The listing builds one solid part. Answer for the finished solid, in the listing's coordinates (mm). Face numbers are marked on the shaded views. A direction names the side the tool comes from. Coordinates: 2 decimals unless noted, no trailing zeros. Order: outer loops, then holes, each group sorted by start corner. A loop starts at its lowest first (then second) coordinate and runs counter-clockwise, first axis right, second up. Notation, with made-up numbers: M -6,43.5 L 1,43.5 A30 ccw 1,80.5 Z; hole C -20.75,6 d5. An arc over 180 degrees is marked long. One line per item, written item: value. Start each with the question number.
Q1. The part is cut by section C-C on y = 13.5. Give the vertices of the cut face in (x, z), then the cut area to 3 significant figures.
Q2. The part is cut by section A-A on z = -27. Give the vertices of the cut face in (x, y) (3 decimals), then the cut area to 3 significant figures.
Q3. Each of these flat-tipped pins is pushed along its axis until it touches: pin 1 Ø3 at (x, z) = (-5, -5) entering from +Y; pin 2 Ø3.5 at (y, z) = (7, -26) entering from +X; pin 3 Ø1.5 at (y, z) = (4.5, -25) entering from -X; pin 4 Ø7 at (x, z) = (-4.5, -21) entering from +Y. Where does it stop, or does it pass through?
Q4. Determine the mould class of the marked faces 1, 2, 3 and 4 for opening direction X: pulls with the +X half, pulls with the -X half, needs draft (parallel to the pull), parting line crosses it, or undercut.
Q5. For the marked faces 5, 6 and 7, determine the directions among +Z, -Z, +X, -X, +Y, -Y from which every point of the face is accessible in a straight line to the end or side of a thin tool.
Q6. The part is cut by section B-B on x = -5. Give the vertices of the cut face in (y, z), then the cut area to 3 significant figures.
Q7. Straight lines are drawn through the part: line 1 along Z through (x, y) = (-43, 1.1); line 2 along X through (y, z) = (13.25, -19.5); line 3 along X through (y, z) = (1.25, -30). For each, find the intervals that lie inside material, in ascending order. Write a range as [from, to].
Q8. The part is cut by section D-D on z = -5. Give the vertices of the cut face in (x, y), then the cut area to 3 significant figures.
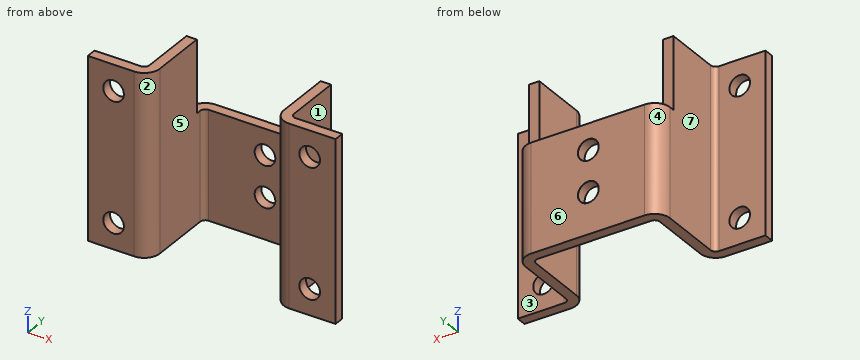
```python
from build123d import *

# Parameters (mm, degrees)
BASE_FLANGE1_DEPTH                 = 35
SKETCH6_W                          = 28
SKETCH6_H                          = 14
CUT_EXTRUDE1_DEPTH                 = 4
F_4_0_4_DIAMETER_HOLE1_D           = 4
F_4_0_4_DIAMETER_HOLE1_CSINK_D     = 4.05
F_4_0_4_DIAMETER_HOLE1_CSINK_ANGLE = 90


# Sheet-metal steps are written as plain solids
with BuildPart() as part:
    # Sketch1 → Base-Flange1 (new body)
    with BuildSketch(Plane.XY):
        with BuildLine():
            Line((0, 0), (-9, 0))
            ThreePointArc((-9, 0), (-11.121320344, 0.878679656), (-12, 3))
            Line((-12, 3), (-12, 15))
            ThreePointArc((-12, 15), (-12.292893219, 15.707106781), (-13, 16))
            Line((-13, 16), (-35, 16))
            ThreePointArc((-35, 16), (-35.707106781, 15.707106781), (-36, 15))
            Line((-36, 15), (-36, 3))
            ThreePointArc((-36, 3), (-36.878679656, 0.878679656), (-39, 0))
            Line((-39, 0), (-48, 0))
            Line((-48, 0), (-48, 2))
            Line((-48, 2), (-39, 2))
            ThreePointArc((-39, 2), (-38.292893219, 2.292893219), (-38, 3))
            Line((-38, 3), (-38, 15))
            ThreePointArc((-38, 15), (-37.121320344, 17.121320344), (-35, 18))
            Line((-35, 18), (-13, 18))
            ThreePointArc((-13, 18), (-10.878679656, 17.121320344), (-10, 15))
            Line((-10, 15), (-10, 3))
            ThreePointArc((-10, 3), (-9.707106781, 2.292893219), (-9, 2))
            Line((-9, 2), (0, 2))
            Line((0, 2), (0, 0))
        make_face()
    extrude(amount=-BASE_FLANGE1_DEPTH)

    # Sketch6 → Cut-Extrude1 (cut)
    with BuildSketch(Plane(origin=(0, 18, 0), x_dir=(1, 0, 0), z_dir=(0, 1, 0))):
        with Locations((-24, 7)):
            Rectangle(SKETCH6_W, SKETCH6_H)
    extrude(amount=-CUT_EXTRUDE1_DEPTH, mode=Mode.SUBTRACT)

    # Ø4.0 (4) Diameter Hole1 (through all)
    with Locations(Plane(origin=(0, 18, 0), x_dir=(1, 0, 0), z_dir=(0, 1, 0))):
        with Locations((-24.099356194, 27), (-24.099356194, 19), (-43, 30), (-43, 5), (-5, 5), (-5, 30)):
            CounterSinkHole(F_4_0_4_DIAMETER_HOLE1_D / 2, F_4_0_4_DIAMETER_HOLE1_CSINK_D / 2, counter_sink_angle=F_4_0_4_DIAMETER_HOLE1_CSINK_ANGLE)


solid = part.part
```
Output:
1. outline: M -38,-35 L -36,-35 L -36,0 L -38,0 Z; M -12,-35 L -10,-35 L -10,0 L -12,0 Z
1. area: 140 mm^2
2. outline: M -48,0 L -39,0 A3 ccw -36,3 L -36,15 A1 cw -35,16 L -26.099,16 L -26.099,17.975 L -26.124,18 L -35,18 A3 ccw -38,15 L -38,3 A1 cw -39,2 L -48,2 Z; M -22.099,16 L -13,16 A1 cw -12,15 L -12,3 A3 ccw -9,0 L 0,0 L 0,2 L -9,2 A1 cw -10,3 L -10,15 A3 ccw -13,18 L -22.074,18 L -22.099,17.975 Z
2. area: 145 mm^2
3. pin 1: passes through
3. pin 2: stops at x = -10
3. pin 3: stops at x = -38
3. pin 4: stops at y = 2
4. face 1: pulls with the +X half
4. face 2: undercut
4. face 3: needs draft
4. face 4: pulls with the -X half
5. face 5: +Z, -Z, -Y
5. face 6: +Z, -Z, +X, -X, +Y
5. face 7: +Z, -Z, -X, +Y
6. outline: M 0,-35 L 2,-35 L 2,-32 L 0,-32 Z; M 0,-28 L 2,-28 L 2,-7 L 0,-7 Z; M 0,-3 L 2,-3 L 2,0 L 0,0 Z
6. area: 54.0 mm^2
7. line 1: z = [-35, -32], [-28, -7], [-3, 0]
7. line 2: x = [-38, -36], [-12, -10]
7. line 3: x = [-48, -45], [-41, -36.56], [-11.44, -7], [-3, 0]
8. outline: M -48,0 L -45,0 L -45,2 L -48,2 Z; M -41,0 L -39,0 A3 ccw -36,3 L -36,14 L -38,14 L -38,3 A1 cw -39,2 L -41,2 Z; M -12,3 A3 ccw -9,0 L -7,0 L -7,2 L -9,2 A1 cw -10,3 L -10,14 L -12,14 Z; M -3,0 L 0,0 L 0,2 L -3,2 Z
8. area: 76.6 mm^2
